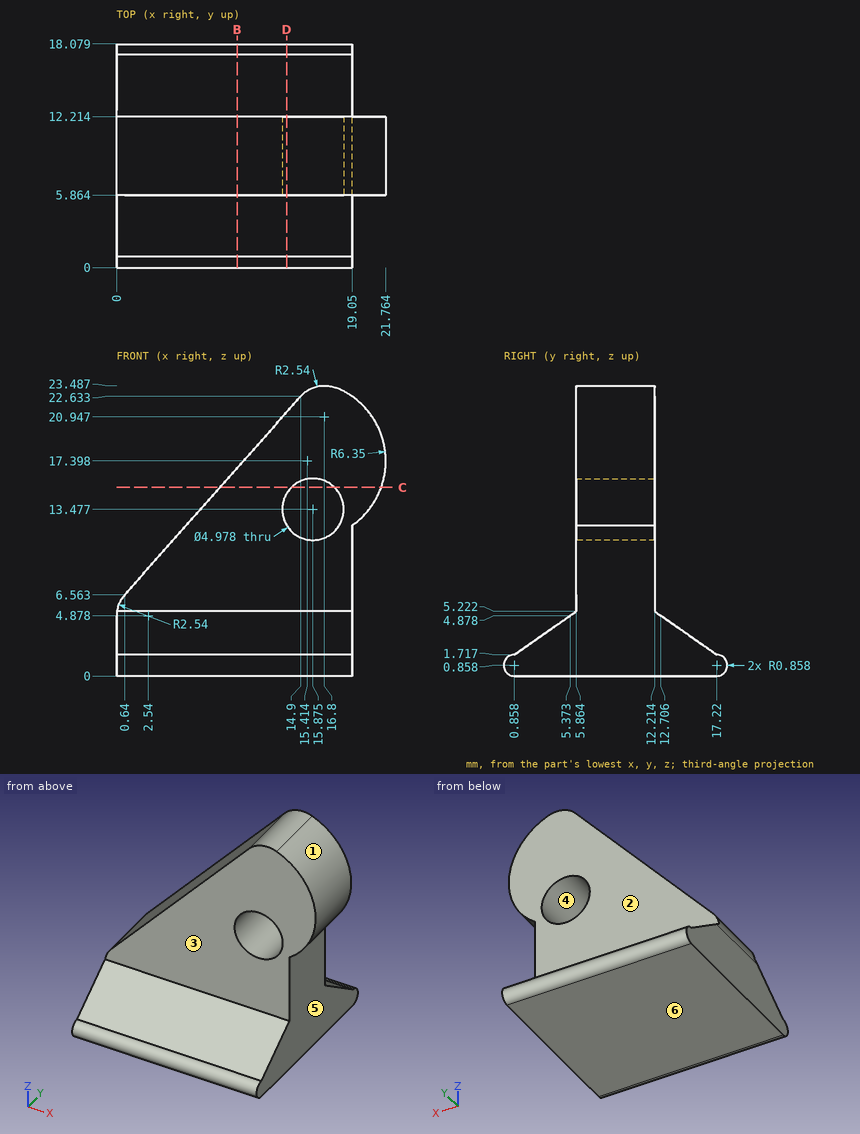
Can you work these out from the drawing? Everything is in mm from the part's minimum corner. A direction names the side the tool comes from. Coordinates: 2 decimals unless noted, no trailing zeros. Write each loop counter-clockwise with the first axis right and the second up, starting at its lowest first coordinate (ties: lowest second). Pieces come first, ordered by that corner, then holes. Notation, with made-up numbers: (86, 41) - (140, 41) arc R21 cw to (140, 63) - close; hole circle Ø9 at (-30.75, 75.25). An arc over 180 degrees is marked (long way). Use a Markdown table: item, result.
Q1. Please list where these lines run through material, in increasing order: L1, parallel to Y at x = 11, z = 7.25 (1 decimal); L2, parallel to Z at x = 15, y = 9 (1 decimal); L3, parallel to X at y = 11.5, z = 3.25.
Geometry check:
| item | result |
|---|---|
| L1 | y = 5.9 to 12.2 |
| L2 | z = 0 to 11.1, 15.8 to 22.7 |
| L3 | x = 0 to 19.05 |
Q2. Thinking about a two-plate mould opening in Z: for the marked faces 4, 5 and 6, which applies, +Z half, -Z half, draft (parallel to the pull), parting line (faces both ways), or undercut?
Geometry check:
| item | result |
|---|---|
| face 4 | undercut |
| face 5 | draft |
| face 6 | -Z half |
Q3. Imagine slicing it at B-B (x = 9.75). List the corners of the cut face in (y, z) for me (1 decimal), and give its area (3 significant figures).
Geometry check:
| item | result |
|---|---|
| outline | (0.9, 0) - (17.2, 0) arc R0.9 ccw to (17.2, 1.7) - (12.2, 5.2) - (12.2, 16.8) - (5.9, 16.8) - (5.9, 5.2) - (0.9, 1.7) arc R0.9 ccw to start |
| area | 144 mm2 |
Q4. Imagine slicing it at C-C (z = 15.25). List the corners of the cut face in (x, y) for me (1 decimal).
Geometry check:
| item | result |
|---|---|
| outline | (8.3, 5.9) - (14.1, 5.9) - (14.1, 12.2) - (8.3, 12.2) - close; (17.6, 5.9) - (21.4, 5.9) - (21.4, 12.2) - (17.6, 12.2) - close |
Q5. Imagine slicing it at D-D (x = 13.75). List the corners of the cut face in (y, z) for me (1 decimal).
Geometry check:
| item | result |
|---|---|
| outline | (0.9, 0) - (17.2, 0) arc R0.9 ccw to (17.2, 1.7) - (12.2, 5.2) - (12.2, 12.2) - (5.9, 12.2) - (5.9, 5.2) - (0.9, 1.7) arc R0.9 ccw to start; (5.9, 14.8) - (12.2, 14.8) - (12.2, 21.3) - (5.9, 21.3) - close |
Q6. I'm going to push flat-ended pins straight in: pin 1 Ø5.5 at (x, z) = (6.5, 15) entering from +Y; pin 2 Ø5 at (x, y) = (9.5, 13) entering from +Z; pin 3 Ø8 at (y, z) = (11.5, 13) entering from -X; pin 4 Ø3 at (x, z) = (15.88, 13.48) entering from +Y. Where does each tip first touch, or does it pass through?
Geometry check:
| item | result |
|---|---|
| pin 1 | stops at y = 12.21 |
| pin 2 | stops at z = 19.22 |
| pin 3 | stops at x = 2.8 |
| pin 4 | passes through |
Q7. Which directions (+Z, -Z, +X, -X, +Y, -Y) give clear straight access to the entire face, cutting with the end or side of a thin tool? Please do the marked faces 1, 2 and 3.
Geometry check:
| item | result |
|---|---|
| face 1 | +X, +Y, -Y |
| face 2 | +Z, +X, -X, +Y |
| face 3 | +Z, +X, -X, -Y |
